The listing builds one solid part. Answer for the finished solid, in the listing's coordinates (mm). A direction names the side the tool comes from. Round coordinates to 2 decimals unless told otherwise and drop trailing zeros. Write each loop counter-clockwise with the first axis right and the second up, starting at its lowest first coordinate (ties: lowest second). Pieces come first, ordered by that corner, then holes. Notation, with made-up numbers: (42.25, 69) - (95.25, 69) arc R33 cw to (95.25, 97) - close; hole circle Ø2 at (-2, 38.5). An arc over 180 degrees is marked (long way). Return JSON: item names as keys, results as strings. Group by question number.
from build123d import *

# Parameters (mm, degrees)
SKETCH_2_R          = 42
SKETCH_2_R_2        = 1
EXTRUDE_1_DEPTH     = 5
SKETCH_3_R          = 1
EXTRUDE_2_DEPTH     = 5
SKETCH_4_R          = 5
CUT_EXTRUDE_1_DEPTH = 5
SKETCH_5_W          = 3
SKETCH_5_H          = 6.5
CUT_EXTRUDE_2_DEPTH = 5


with BuildPart() as part:
    # 草图2 → 凸台-拉伸1 (new body)
    # profile 1 of 2: a face of its own
    with BuildSketch(Plane.XY):
        Circle(SKETCH_2_R)
        with Locations((0, 40)):
            Circle(SKETCH_2_R_2, mode=Mode.SUBTRACT)
    # profile 2 of 2: a face of its own
    with BuildSketch(Plane.XY):
        with Locations((0, 40)):
            Circle(SKETCH_2_R_2)
    extrude(amount=EXTRUDE_1_DEPTH)

    # 草图3 → 凸台-拉伸2 (add)
    with BuildSketch(Plane.XY.offset(5)):
        with Locations((0, 40)):
            Circle(SKETCH_3_R)
    extrude(amount=EXTRUDE_2_DEPTH)

    # 草图4 → 切除-拉伸1 (cut)
    with BuildSketch(Plane.XY.offset(5)):
        Circle(SKETCH_4_R)
    extrude(amount=-CUT_EXTRUDE_1_DEPTH, mode=Mode.SUBTRACT)

    # 草图5 → 切除-拉伸2 (cut)
    with BuildSketch(Plane.XY.offset(5)):
        with Locations((0, 3.25)):
            Rectangle(SKETCH_5_W, SKETCH_5_H)
    extrude(amount=-CUT_EXTRUDE_2_DEPTH, mode=Mode.SUBTRACT)


solid = part.part
(1) Consider line 1 (Y direction, x = 0, z = 1.25); line 2 (Z direction, x = 16, y = 17.5); line 3 (Y direction, x = 12.5, z = 4). Determine where each line is inside the solid, lowest interval first.
(2) For faces 1 (the cylindrical face through (0, 41, 7)), 2 (the flat face through (0, 6.5, 3)), 3 (the flat face through (9, 1, 0)), determine the directions among +Z, -Z, +X, -X, +Y, -Y from which every point of the face is accessible in a straight line to the end or side of a thin tool.
(3) Find section D-D (z = 6.25). Write down the section's boundary in (x, y).
(4) Flat-ended cylindrical pins translate along their axes: pin 1 (1.4 mm diameter, centred on y = 5.5, z = 1.5, fed in from +X); pin 2 (1 mm diameter, centred on x = -17, y = -28.5, fed in from +Z); pin 3 (1.4 mm diameter, centred on y = 5.5, z = 1.5, fed in from -X). Find the tip coordinate at first contact, or state that the pin passes through.
(5) Find section C-C (y = 40). Write down the section's boundary in (x, z), plus the area to 3 significant figures.
(6) Find section B-B (x = 0). Write down the section's boundary in (y, z).
(7) Determine the mould class of faces 4 (the flat face through (0, 40, 10)), 5 (the cylindrical face through (0, -5, 3)), 6 (the cylindrical face through (40.06, 12.62, 2.46)) for opening direction X: +X half, -X half, draft (parallel to the pull), parting line (faces both ways), or undercut.
(8) Find section A-A (y = 0). Write down the section's boundary in (x, z).
Check sheet entries:
{
 "1": {"line 1": "y = -42 to -5, 6.5 to 42", "line 2": "z = 0 to 5", "line 3": "y = -40.1 to 40.1"},
 "2": {"face 1": "+Z", "face 2": "+Z, -Z", "face 3": "-Z, +X, -X, +Y, -Y"},
 "3": {"outline": "circle Ø2 at (0, 40)"},
 "4": {"pin 1": "stops at x = 41.72", "pin 2": "stops at z = 5", "pin 3": "stops at x = -41.72"},
 "5": {"outline": "(-12.81, 0) - (12.81, 0) - (12.81, 5) - (1, 5) - (1, 10) - (-1, 10) - (-1, 5) - (-12.81, 5) - close", "area": "138 mm^2"},
 "6": {"outline": "(-42, 0) - (-5, 0) - (-5, 5) - (-42, 5) - close; (6.5, 0) - (42, 0) - (42, 5) - (41, 5) - (41, 10) - (39, 10) - (39, 5) - (6.5, 5) - close"},
 "7": {"face 4": "draft", "face 5": "undercut", "face 6": "parting line"},
 "8": {"outline": "(-42, 0) - (-5, 0) - (-5, 5) - (-42, 5) - close; (5, 0) - (42, 0) - (42, 5) - (5, 5) - close"}
}
